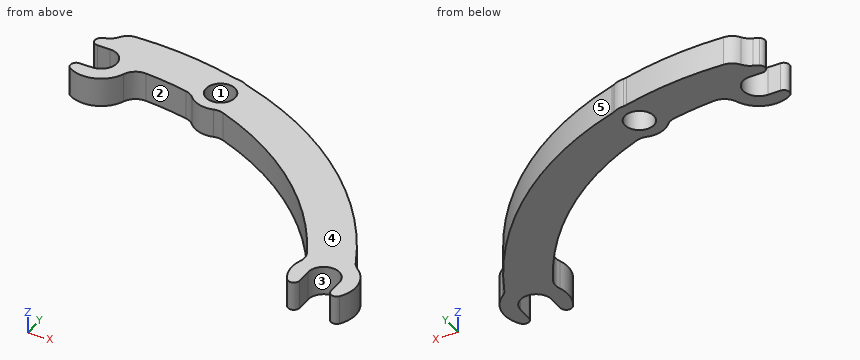
Autodesk Inventor part; units mm, degrees
ref_plane "YZ Plane" through (0, 0, 0) normal (1, 0, 0) x (0, 1, 0)
ref_plane "XZ Plane" through (0, 0, 0) normal (0, 1, 0) x (-1, 0, 0)
ref_plane "XY Plane" through (0, 0, 0) normal (0, 0, 1) x (1, 0, 0)
sketch "Sketch1" plane through (0, 0, 0) normal (0, 0, 1) x (1, 0, 0)
  line L0 (0, 0) -> (69.8506, 0) construction
  circle A0 centre (0, -41.91) radius 47.625 construction
  arc A1 (0, -1.7145) -> (0, 1.7145) centre (0, 0) ccw
  arc A2 (-2.896, -1.7145) -> (-2.896, 1.7145) centre (0, 0) ccw
  line L1 (0, 3.3655) -> (0, 4.6355)
  arc A3 (38.0096, -20.955) -> (34.5806, -20.955) centre (36.2951, -20.955) ccw
  arc A4 (38.0096, -23.9977) -> (34.5806, -23.9977) centre (36.2951, -20.955) ccw
  arc A5 (38.0096, -17.9123) -> (0, 4.6355) centre (2.7126, -34.1027) ccw
  arc A6 (33.341, -19.092) -> (3.3655, 0) centre (2.7126, -34.1027) ccw
  line L2 (0, 1.7145) -> (-2.896, 1.7145)
  line L3 (0, -1.7145) -> (-2.896, -1.7145)
  line L4 (34.5806, -20.955) -> (34.5806, -23.9977)
  line L5 (38.0096, -20.955) -> (38.0096, -23.9977)
  dimension "d0" = 41.91
  dimension "d2" = 30
  dimension "d3" = 95.25
  dimension "d4" = 41.91
  dimension "d5" = 41.91
  dimension "d6" = 3.429
  dimension "d7" = 6.731
  dimension "d8" = 1.27
  dimension "d9" = 3.429
  dimension "d10" = 6.985
extrude "Extrusion1" add sketch "Sketch1" along normal blind 3.175
fillet "Fillet1" radius 0.635 4 edges at (-2.896, -1.7145, 1.5875) (-2.896, 1.7145, 1.5875) (34.5806, -23.9977, 1.5875) (38.0096, -23.9977, 1.5875)
fillet "Fillet2" radius 1.778 5 edges at (0, 3.3655, 1.5875) (0, 4.6355, 1.5875) (3.3655, 0, 1.5875) (33.341, -19.092, 1.5875) (38.0096, -17.9123, 1.5875)
sketch "Sketch2" plane through (0, 0, 3.175) normal (0, 0, 1) x (1, 0, 0)
  circle A0 centre (12.7, 0.635) radius 1.5875
  point P0 (0, 0)
  dimension "d15" = 3.175
  dimension "d16" = 12.7
  dimension "d17" = 0.635
extrude "Extrusion2" cut sketch "Sketch2" against normal through all
sketch "Sketch3" plane through (0, 0, 3.175) normal (0, 0, 1) x (1, 0, 0)
  circle A0 centre (12.7, 0.635) radius 1.5875
  circle A1 centre (12.7, 0.635) radius 2.794
  point P0 (0, 0)
  dimension "d20" = 5.588
extrude "Extrusion3" add sketch "Sketch3" against normal blind 3.175
fillet "Fillet3" radius 1.778 4 edges at (14.1994, 2.9926, 1.5875) (12.6817, 3.4289, 1.5875) (13.9092, -1.8838, 1.5875) (10.3377, -0.857, 1.5875)
properties part number "HallEffectSpoolSensorMount3Brace" material "ABS Plastic"
The listing builds one solid part. Answer for the finished solid, in the listing's coordinates (mm). Face numbers are marked on the shaded views. A direction names the side the tool comes from. Round coordinates to 2 decimals unless told otherwise and drop trailing zeros. Write each loop counter-clockwise with the first axis right and the second up, starting at its lowest first coordinate (ties: lowest second). Pieces come first, ordered by that corner, then holes. Notation, with made-up numbers: M -19,83 L 6,83 A32 ccw 6,121 Z; hole C 16,-3.5 d3. An arc over 180 degrees is marked long. Write each question's results on one line, items separated by ' | '. Start each with the question number.
Item 1: Given pin 1 Ø1 at (y, z) = (-1, 2) entering from +X; pin 2 Ø0.8 at (y, z) = (-22, 1) entering from -X; pin 3 Ø0.8 at (y, z) = (-21.5, 2.5) entering from +X, each flat-ended and moving along its own axis, determine where each tip first touches the part or whether it passes through.
Item 2: The mould has two halves that part along X. Classify the marked faces 3, 4 and 5: +X half, -X half, draft (parallel to the pull), parting line (faces both ways), or undercut.
Item 3: Straight lines are drawn through the part: probe 1 along X at (y, z) = (-19.75, 1.5); probe 2 along Y at (x, z) = (12.7, 2.35); probe 3 along X at (y, z) = (-21.25, 0.5). For each, find the intervals that lie inside material, in ascending order.
Item 4: Find section A-A on y = -14. Write down the section's boundary in (x, z) (3 decimals).
Item 5: Which of the six approach directions +Z, -Z, +X, -X, +Y, -Y give full straight-line access (tool end or side, diameter ignored) to the marked faces 1 and 2?
Item 6: Find section B-B on x = 18.5. Write down the section's boundary in (y, z) (3 decimals), and give its area (3 significant figures).
Answer block:
1) pin 1: stops at x = 23.81 | pin 2: stops at x = 32.86 | pin 3: stops at x = 39.78
2) face 3: undercut | face 4: draft | face 5: +X half
3) probe 1: x = 33.02 to 35.08, 37.51 to 39.57 | probe 2: y = -2.16 to -0.95, 2.22 to 3.44 | probe 3: x = 32.82 to 34.58, 38.01 to 39.78
4) outline: M 30.268,0 L 35.937,0 L 35.937,3.175 L 30.268,3.175 Z
5) face 1: +Z, -Z | face 2: +Z, -Z, -Y
6) outline: M -3.867,0 L 1.376,0 L 1.376,3.175 L -3.867,3.175 Z | area: 16.6 mm²
